```python
from build123d import *

# Parameters (mm, degrees)
BODY_SKETCH_R    = 25.4
WHEEL_BODY_DEPTH = 9.525
FILLET_WHEEL_R   = 1
HOLE_SKETCH_R    = 2.305
HOLE_SHAFT_DEPTH = 15


with BuildPart() as part:
    # body sketch → wheel body (new, symmetric)
    with BuildSketch(Plane.XY):
        with Locations(Location((0, 0, 0), (0, 0, 180))):
            Circle(BODY_SKETCH_R)
    extrude(amount=WHEEL_BODY_DEPTH, both=True)

    # fillet wheel
    fillet_wheel_edges = [part.edges().sort_by_distance(p)[0] for p in [
        (25.4, 0, -9.525),
        (25.4, 0, 9.525),
    ]]
    fillet(fillet_wheel_edges, radius=FILLET_WHEEL_R)

    # hole sketch → hole shaft (cut)
    with BuildSketch(Plane.XY.offset(9.525)):
        Circle(HOLE_SKETCH_R)
    extrude(amount=-HOLE_SHAFT_DEPTH, mode=Mode.SUBTRACT)


solid = part.part
```
The listing builds one solid part. Answer for the finished solid, in the listing's coordinates (mm). Coordinates: 2 decimals unless noted, no trailing zeros. Loops run counter-clockwise (first coordinate to the right, second up) from the corner with the lowest first, then second, coordinate; pieces in that order, holes last. Notation, with made-up numbers: (86, 37) - (103, 37) arc R15 cw to (103, 44) - close; hole circle Ø9 at (85, 35.5). An arc over 180 degrees is marked (long way). Use a Markdown table: item, result. Add a question column.
1) Find the intervals of material crossed by line 1 (Y direction, x = 0, z = 3.75) (3 decimals); line 2 (X direction, y = -11.5, z = -8.5); line 3 (X direction, y = -20, z = -5), in increasing order.
2) Given pin 1 (5 mm diameter, centred on x = 15, z = -2.5, fed in from -Y); pin 2 (5 mm diameter, centred on y = 18, z = 5.5, fed in from +X); pin 3 (8 mm diameter, centred on x = -15, z = -6.5, fed in from +Y), each flat-ended and moving along its own axis, determine where each tip first touches the part or whether it passes through.
3) The mould has two halves that part along Y. Classify faces 1 (the cylindrical face through (-11.721, 22.534, 0.119)), 2 (the cylindrical face through (2.2, 0.69, 2.13)), 3 (the flat face through (-5, 0, 9.525)), 4 (the flat face through (0, 0, -5.475)): released by +Y, released by -Y, zero draft, split by the parting line, or undercut.
4) The part is cut by section A-A, the plane x = 0. Give the vertices of the cut face in (y, z) (3 decimals), and give its area (3 significant figures).
Here are the results:
| question | item | result |
|---|---|---|
| 1 | line 1 | y = -25.4 to -2.305, 2.305 to 25.4 |
| 1 | line 2 | x = -22.65 to 22.65 |
| 1 | line 3 | x = -15.66 to 15.66 |
| 2 | pin 1 | stops at y = -22.11 |
| 2 | pin 2 | stops at x = 20.12 |
| 2 | pin 3 | stops at y = 22.89 |
| 3 | face 1 | split by the parting line |
| 3 | face 2 | undercut |
| 3 | face 3 | zero draft |
| 3 | face 4 | undercut |
| 4 | outline | (-25.4, -8.525) arc R1 ccw to (-24.4, -9.525) - (24.4, -9.525) arc R1 ccw to (25.4, -8.525) - (25.4, 8.525) arc R1 ccw to (24.4, 9.525) - (2.305, 9.525) - (2.305, -5.475) - (-2.305, -5.475) - (-2.305, 9.525) - (-24.4, 9.525) arc R1 ccw to (-25.4, 8.525) - close |
| 4 | area | 898 mm^2 |
